```python
from build123d import *

# Parameters (mm, degrees)
SHELL1_T           = -1
CUT_EXTRUDE1_REACH = 272.851


with BuildPart() as part:
    # Sketch1 → Revolve1 (revolve)
    with BuildSketch(Plane.XY, mode=Mode.PRIVATE) as revolve1_sk:
        Polygon((0, 0), (109.979208013, 0), (109.161205132, 24.375928632), (107.208857797, 24.375928632), (107.208857797, 26.816923755), (109.079290671, 26.816923755), (106.752331603, 96.158718868), (104.799984268, 96.158718868), (104.799984268, 98.599713991), (106.670417142, 98.599713991), (106.0385402, 117.429216448), (0, 117.429216448), align=None)
    revolve(revolve1_sk.sketch.rotate(Axis((0, 117.429216448, 0), (0, -1, 0)), 90), axis=Axis((0, 117.429216448, 0), (0, -1, 0)))

    # Shell1
    shell1_openings = [part.faces().sort_by_distance(p)[0] for p in [
        (0, 0, 0),
        (0, 117.429216448, 0),
    ]]
    offset(amount=SHELL1_T, openings=shell1_openings, kind=Kind.INTERSECTION)

    # Sketch2 → Cut-Extrude1 (cut, up to next)
    with BuildSketch(Plane(origin=(109.855496784, 3.686510337, 0), x_dir=(0, 0, -1), z_dir=(0.9994374116718343, 0.03353893484749475, 0)), mode=Mode.PRIVATE) as cut_extrude1_sk1:
        with BuildLine():
            Line((-50.869164149, 11.565080514), (49.86916415, 11.565080514))
            ThreePointArc((49.86916415, 11.565080514), (56.940231962, 14.494012702), (59.86916415, 21.565080514))
            Line((59.86916415, 21.565080514), (59.86916415, 89.360085428))
            ThreePointArc((59.86916415, 89.360085428), (56.940231962, 96.43115324), (49.86916415, 99.360085428))
            Line((49.86916415, 99.360085428), (-50.869164149, 99.360085428))
            ThreePointArc((-50.869164149, 99.360085428), (-57.940231961, 96.43115324), (-60.869164149, 89.360085428))
            Line((-60.869164149, 89.360085428), (-60.869164149, 21.565080514))
            ThreePointArc((-60.869164149, 21.565080514), (-57.940231961, 14.494012702), (-50.869164149, 11.565080514))
        make_face()
    cut_extrude1_tool1 = extrude(cut_extrude1_sk1.sketch, amount=-CUT_EXTRUDE1_REACH, mode=Mode.PRIVATE) & part.part
    add(cut_extrude1_tool1.solids().sort_by_distance((107.995341, 59.117891, 0.5))[0], mode=Mode.SUBTRACT)


solid = part.part
```
Read the model definition and answer for the solid it produces. Units are mm, in the model's axes. A direction names the side the tool comes from. Round coordinates to 2 decimals unless told otherwise and drop trailing zeros. Write each loop counter-clockwise with the first axis right and the second up, starting at its lowest first coordinate (ties: lowest second). Pieces come first, ordered by that corner, then holes. Notation, with made-up numbers: (76.25, -0.75) -> (86.25, -0.75) arc R15 cw to (86.25, 20.25) -> close; hole circle Ø9 at (-31.5, 10.25). An arc over 180 degrees is marked (long way). Answer in a Markdown table with one row per item. Add a question column.
1) Determine the mould class of faces 4 (the face through (20, 27.817, 105)), 5 (the face through (-24, 117.429, -103)), 6 (the face through (-88.3, 95.159, -55.3)) for opening direction Y: pulls with the +Y half, pulls with the -Y half, needs draft (parallel to the pull), parting line crosses it, or undercut.
2) Given P1, Ø12, axis at x = -27, y = 59.5, coming from the -Z side; P2, Ø5, axis at x = -68, y = 101, coming from the -Z side; P3, Ø5, axis at x = 66, z = -80.5, coming from the +Y side; P4, Ø2, axis at y = 24, z = 84.5, coming from the +X side, each flat-ended and moving along its own axis, determine where each tip first touches the part or whether it passes through.
3) Find section C-C, the plane y = 39.5. Determine the outline of the cut face in (x, z), and give its area (3 significant figures).
4) Find section B-B, the plane y = 73. Determine the outline of the cut face in (x, z).
5) Consider line 1 (Z direction, x = 0, y = 97.55); line 2 (Z direction, x = 0, y = 26); line 3 (X direction, y = 97, z = 0). Determine where each line is inside the solid, lowest interval first.
6) Which of the six approach directions +Z, -Z, +X, -X, +Y, -Y give full straight-line access (tool end or side, diameter ignored) to faces 1 (the face through (-106.16, 25.63, 3.16)), 2 (the face through (-105.306, 112.331, -13.826)), 3 (the face through (-106.85, 61.96, 3.22))?
Findings below:
| question | item | result |
|---|---|---|
| 1 | face 4 | undercut |
| 1 | face 5 | pulls with the +Y half |
| 1 | face 6 | pulls with the -Y half |
| 2 | P1 | z = -105.94 |
| 2 | P2 | z = -84.09 |
| 2 | P3 | y = 117.43 |
| 2 | P4 | x = 70.33 |
| 3 | outline | (88.79, 60.87) -> (90, 60.87) arc R108.65 ccw (long way) to (90.67, -59.87) -> (89.47, -59.87) arc R107.65 cw (long way) to start |
| 3 | area | 552 mm² |
| 4 | outline | (87.43, 60.87) -> (88.64, 60.87) arc R107.53 ccw (long way) to (89.32, -59.87) -> (88.11, -59.87) arc R106.53 cw (long way) to start |
| 5 | line 1 | -104.8 to -103.8, 103.8 to 104.8 |
| 5 | line 2 | -107.21 to -106.21, 106.21 to 107.21 |
| 5 | line 3 | -104.8 to -103.8 |
| 6 | face 1 | -Y |
| 6 | face 2 | +Y |
| 6 | face 3 | none |
